Check sheet for the modelled part. Datum: model origin and axes. Units: mm. Give positions to 0.01 mm unless a question says otherwise; leave off trailing zeros. Order: outer loops, then holes, each group sorted by start corner. A loop starts at its lowest first (then second) coordinate and runs counter-clockwise, first axis right, second up.
from build123d import *

# Parameters (mm, degrees)
SKETCH1_W                                           = 32
SKETCH1_H                                           = 32
BOSS_EXTRUDE1_DEPTH                                 = 7
CSK_FOR_M6_COUNTERSUNK_FLAT_HEAD_SCREW2_D           = 6
CSK_FOR_M6_COUNTERSUNK_FLAT_HEAD_SCREW2_DEPTH       = 23
CSK_FOR_M6_COUNTERSUNK_FLAT_HEAD_SCREW2_CSINK_D     = 13
CSK_FOR_M6_COUNTERSUNK_FLAT_HEAD_SCREW2_CSINK_ANGLE = 90
CSK_FOR_M6_COUNTERSUNK_FLAT_HEAD_SCREW2_TIP         = 1.802581857


with BuildPart() as part:
    # Sketch1 → Boss-Extrude1 (new body)
    with BuildSketch(Plane.XY):
        with Locations((38.880175665, -11.244087205)):
            Rectangle(SKETCH1_W, SKETCH1_H)
    extrude(amount=BOSS_EXTRUDE1_DEPTH)

    # CSK for M6 Countersunk Flat Head Screw2
    with Locations(Plane.XY.offset(7)):
        with Locations((30.880175665, -11.244087205), (46.880175665, -11.244087205)):
            CounterSinkHole(CSK_FOR_M6_COUNTERSUNK_FLAT_HEAD_SCREW2_D / 2, CSK_FOR_M6_COUNTERSUNK_FLAT_HEAD_SCREW2_CSINK_D / 2, depth=CSK_FOR_M6_COUNTERSUNK_FLAT_HEAD_SCREW2_DEPTH, counter_sink_angle=CSK_FOR_M6_COUNTERSUNK_FLAT_HEAD_SCREW2_CSINK_ANGLE)
            with Locations((0, 0, -(CSK_FOR_M6_COUNTERSUNK_FLAT_HEAD_SCREW2_DEPTH + CSK_FOR_M6_COUNTERSUNK_FLAT_HEAD_SCREW2_TIP / 2))):  # 118° drill point
                Cone(0, CSK_FOR_M6_COUNTERSUNK_FLAT_HEAD_SCREW2_D / 2, CSK_FOR_M6_COUNTERSUNK_FLAT_HEAD_SCREW2_TIP, mode=Mode.SUBTRACT)


solid = part.part
1) Material ranges on L1, parallel to X at y = -14, z = 6.5; L2, parallel to X at y = -14, z = 1; L3, parallel to Y at x = 31, z = 1.5, recorded low to high.
Recorded:
L1: x = 22.88 to 25.55, 36.21 to 41.55, 52.21 to 54.88
L2: x = 22.88 to 29.69, 32.07 to 45.69, 48.07 to 54.88
L3: y = -27.24 to -14.24, -8.25 to 4.76
2) Draft check along X on faces 1 (the face through (33.877, -11.112, 1.726)), 2 (the face through (54.88, -11, 3)), 3 (the face through (39, 4.756, 3)). Enter one of: +X half, -X half, draft (parallel to the pull), parting line (faces both ways), or undercut.
Recorded:
face 1: undercut
face 2: +X half
face 3: draft
3) Section check B-B, the plane y = -9. State how many separate pieces and enclosed holes the cut face has, then the cut area to 3 significant figures.
Recorded:
separate pieces: 3
enclosed holes: 0
area: 138 mm2
4) Section check A-A, the plane z = 5.75. Record the cut outline in (x, y), then the cut area to 3 significant figures.
Recorded:
outline: (22.88, -27.24) - (54.88, -27.24) - (54.88, 4.76) - (22.88, 4.76) - close; hole circle Ø10.5 at (30.88, -11.24); hole circle Ø10.5 at (46.88, -11.24)
area: 851 mm2
5) Depth check by flat-ended pin: pin 1 Ø1.5 at (x, y) = (37, -8.5) entering from -Z. Enter the tip coordinate at first touch or a pass-through.
Recorded:
pin 1: stops at z = 0
